```python
from build123d import *

# Parameters (mm, degrees)
SKETCH_1_W      = 300
SKETCH_1_H      = 300
EXTRUDE_1_DEPTH = 300
SHELL_1_T       = -11
SKETCH_3_W      = 300
SKETCH_3_H      = 11
EXTRUDE_2_DEPTH = 300


with BuildPart() as part:
    # 草图1 → 凸台-拉伸1 (new body)
    with BuildSketch(Plane(origin=(0, 0, 0), x_dir=(1, 0, 0), z_dir=(0, 1, 0))):
        Rectangle(SKETCH_1_W, SKETCH_1_H)
    extrude(amount=EXTRUDE_1_DEPTH)

    # 抽壳1
    shell_1_openings = [part.faces().sort_by_distance(p)[0] for p in [
        (0, 150, 150),
    ]]
    offset(amount=SHELL_1_T, openings=shell_1_openings, kind=Kind.INTERSECTION)

    # 草图3 → 凸台-拉伸2 (add)
    with BuildSketch(Plane.XY.offset(150)):
        with Locations((0, 79.5)):
            Rectangle(SKETCH_3_W, SKETCH_3_H)
    extrude(amount=-EXTRUDE_2_DEPTH)


solid = part.part
```
Verification items for the finished model (mm, model axes). A direction names the side the tool comes from. Give positions to 0.01 mm unless a question says otherwise; leave off trailing zeros. Loops run counter-clockwise (first coordinate to the right, second up) from the corner with the lowest first, then second, coordinate; pieces in that order, holes last.
1. Mould release check, pull along X, two halves, no side actions. Record for faces 3 (the flat face through (-150, 148, 2)), 4 (the flat face through (-1, 83, 150)), 5 (the flat face through (-2, 85, 8)), 6 (the flat face through (-2, 42, -139)): released by +X, released by -X, zero draft, split by the parting line, or undercut.
2. Section check C-C, the plane x = -75. Enter the section's corners in (y, z), then the cut area to 3 significant figures.
3. Go/stop test with a flat-tipped pin: pin 1 Ø19 at (x, y) = (-47.5, 57.5) entering from +Z. Record where the tip stops, or that it passes through.
4. Set-up check for faces 1 (the flat face through (150, 148, 2)), 2 (the flat face through (139, 42, 8)): record each of +Z, -Z, +X, -X, +Y, -Y from which the full face is reachable in a straight line by a thin tool's end or side.
5. Thickness scan on line 1 (Y direction, x = 84, z = 108); line 2 (X direction, y = 178, z = 96.5); line 3 (Z direction, x = 94.5, y = 199). Record the ranges inside material, lowest first.
6. Section check A-A, the plane z = 80. Enter the section's corners in (x, y), then the cut area to 3 significant figures.
7. Section check B-B, the plane y = 250.5. Enter the section's corners in (x, z), then the cut area to 3 significant figures.
Geometry says:
1. face 3: released by -X
1. face 4: zero draft
1. face 5: undercut
1. face 6: undercut
2. outline: (0, -150) - (300, -150) - (300, 150) - (289, 150) - (289, -139) - (85, -139) - (85, 150) - (74, 150) - (74, -139) - (11, -139) - (11, 150) - (0, 150) - close
2. area: 12,800 mm2
3. pin 1: stops at z = -139
4. face 1: +Z, -Z, +X, +Y, -Y
4. face 2: +Z
5. line 1: y = 0 to 11, 74 to 85, 289 to 300
5. line 2: x = -150 to -139, 139 to 150
5. line 3: z = -150 to -139
6. outline: (-150, 0) - (150, 0) - (150, 300) - (-150, 300) - close; hole (-139, 11) - (139, 11) - (139, 74) - (-139, 74) - close; hole (-139, 85) - (139, 85) - (139, 289) - (-139, 289) - close
6. area: 15,800 mm2
7. outline: (-150, -150) - (150, -150) - (150, 150) - (139, 150) - (139, -139) - (-139, -139) - (-139, 150) - (-150, 150) - close
7. area: 9,660 mm2
